Can you work these out from the model? Positions are in its coordinate system, mm. Face numbers are marked on the shaded views. A direction names the side the tool comes from. Give positions to 0.01 mm unless a question says otherwise; leave off trailing zeros. Order: outer loops, then holes, each group sorted by start corner. A loop starts at its lowest first (then second) coordinate and runs counter-clockwise, first axis right, second up.
Item 1: I'm going to push flat-ended pins straight in: pin 1 Ø6 at (x, y) = (63.5, 26.5) entering from -Z; pin 2 Ø10 at (x, y) = (108, 65) entering from +Z; pin 3 Ø10 at (x, y) = (104.5, 45.5) entering from -Z. Where does each tip first touch, or does it pass through?
Item 2: I want a section at C-C, the plane z = -7. Write out the boundary of the cut face in (x, y), then the cut area to 3 significant figures.
Item 3: Which directions (+Z, -Z, +X, -X, +Y, -Y) give clear straight access to the entire face, cutting with the end or side of a thin tool? Please do the marked faces 4, 5, 6, 7 and 8.
Item 4: I want a section at B-B, the plane y = 104.5. Write out the boundary of the cut face in (x, z), then the cut area to 3 significant figures.
Item 5: I want a section at A-A, the plane x = 110. Write out the boundary of the cut face in (y, z).
Item 6: If we mould it in two halves opening along Z, with no side actions, what happens to the marked faces 1, 2 and 3? For each: +Z half, -Z half, draft (parallel to the pull), parting line (faces both ways), or undercut.
Item 7: If I drill on line 1 along Z through (x, y) = (106.5, 78); line 2 along X through (y, z) = (33, -24.5); line 3 along X through (y, z) = (111.5, -23), over which ranges is the centre line in solid material (lowest first)?
```python
from build123d import *

# Parameters (mm, degrees)
BOSS_EXTRUDE1_DEPTH = 100
FILLET1_R           = 20
SKETCH5_W           = 40
SKETCH5_H           = 120
BOSS_EXTRUDE2_DEPTH = 20
SKETCH6_W           = 10
SKETCH6_H           = 30
CUT_EXTRUDE1_DEPTH  = 120
SKETCH7_W           = 100
SKETCH7_H           = 100
BOSS_EXTRUDE3_DEPTH = 2
BOSS_EXTRUDE4_DEPTH = 100
SKETCH11_W          = 0.49
SKETCH11_H          = 2
BOSS_EXTRUDE5_DEPTH = 100
SKETCH12_R          = 7.5
CUT_EXTRUDE2_DEPTH  = 40
SKETCH15_W          = 30
SKETCH15_H          = 50
BOSS_EXTRUDE6_DEPTH = 15
SKETCH16_W          = 15
SKETCH16_H          = 50
CUT_EXTRUDE3_DEPTH  = 10


with BuildPart() as part:
    # Sketch3 → Boss-Extrude1 (new body)
    with BuildSketch(Plane(origin=(0, 0, 0), x_dir=(1, 0, 0), z_dir=(0, 1, 0))):
        Polygon((0, 0), (100, 0), (100, 20), (70, 20), align=None)
    extrude(amount=BOSS_EXTRUDE1_DEPTH)

    # Fillet1
    fillet1_edges = [part.edges().sort_by_distance(p)[0] for p in [
        (70, 50, -20),
    ]]
    fillet(fillet1_edges, radius=FILLET1_R)

    # Sketch5 → Boss-Extrude2 (add)
    with BuildSketch(Plane(origin=(100, 0, 0), x_dir=(0, 0, -1), z_dir=(1, 0, 0))):
        with Locations((9.230478953, 50)):
            Rectangle(SKETCH5_W, SKETCH5_H)
    extrude(amount=BOSS_EXTRUDE2_DEPTH)

    # Sketch6 → Cut-Extrude1 (cut)
    with BuildSketch(Plane(origin=(0, 110, 0), x_dir=(1, 0, 0), z_dir=(0, 1, 0))):
        with Locations((110, 9.230478953)):
            Rectangle(SKETCH6_W, SKETCH6_H)
    extrude(amount=-CUT_EXTRUDE1_DEPTH, mode=Mode.SUBTRACT)

    # Sketch7 → Boss-Extrude3 (add)
    with BuildSketch(Plane.XY):
        with Locations((50, 50)):
            Rectangle(SKETCH7_W, SKETCH7_H)
    extrude(amount=BOSS_EXTRUDE3_DEPTH)

    # Sketch10 → Boss-Extrude4 (add)
    with BuildSketch(Plane(origin=(0, 100, 0), x_dir=(1, 0, 0), z_dir=(0, 1, 0))):
        Polygon((100, -2), (98, -2), (99, -3), align=None)
        Polygon((95.99, -2), (96.99, -3), (97.99, -2), align=None)
        Polygon((93.98, -2), (94.98, -3), (95.98, -2), align=None)
        Polygon((91.97, -2), (92.97, -3), (93.97, -2), align=None)
        Polygon((89.96, -2), (90.96, -3), (91.96, -2), align=None)
        Polygon((87.95, -2), (88.95, -3), (89.95, -2), align=None)
        Polygon((85.94, -2), (86.94, -3), (87.94, -2), align=None)
        Polygon((83.93, -2), (84.93, -3), (85.93, -2), align=None)
        Polygon((81.92, -2), (82.92, -3), (83.92, -2), align=None)
        Polygon((79.91, -2), (80.91, -3), (81.91, -2), align=None)
        Polygon((77.9, -2), (78.9, -3), (79.9, -2), align=None)
        Polygon((75.89, -2), (76.89, -3), (77.89, -2), align=None)
        Polygon((73.88, -2), (74.88, -3), (75.88, -2), align=None)
        Polygon((71.87, -2), (72.87, -3), (73.87, -2), align=None)
        Polygon((69.86, -2), (70.86, -3), (71.86, -2), align=None)
        Polygon((67.85, -2), (68.85, -3), (69.85, -2), align=None)
        Polygon((65.84, -2), (66.84, -3), (67.84, -2), align=None)
        Polygon((63.83, -2), (64.83, -3), (65.83, -2), align=None)
        Polygon((61.82, -2), (62.82, -3), (63.82, -2), align=None)
        Polygon((59.81, -2), (60.81, -3), (61.81, -2), align=None)
        Polygon((57.8, -2), (58.8, -3), (59.8, -2), align=None)
        Polygon((55.79, -2), (56.79, -3), (57.79, -2), align=None)
        Polygon((53.78, -2), (54.78, -3), (55.78, -2), align=None)
        Polygon((51.77, -2), (52.77, -3), (53.77, -2), align=None)
        Polygon((49.76, -2), (50.76, -3), (51.76, -2), align=None)
        Polygon((47.75, -2), (48.75, -3), (49.75, -2), align=None)
        Polygon((45.74, -2), (46.74, -3), (47.74, -2), align=None)
        Polygon((43.73, -2), (44.73, -3), (45.73, -2), align=None)
        Polygon((41.72, -2), (42.72, -3), (43.72, -2), align=None)
        Polygon((39.71, -2), (40.71, -3), (41.71, -2), align=None)
        Polygon((37.7, -2), (38.7, -3), (39.7, -2), align=None)
        Polygon((35.69, -2), (36.69, -3), (37.69, -2), align=None)
        Polygon((33.68, -2), (34.68, -3), (35.68, -2), align=None)
        Polygon((31.67, -2), (32.67, -3), (33.67, -2), align=None)
        Polygon((29.66, -2), (30.66, -3), (31.66, -2), align=None)
        Polygon((27.65, -2), (28.65, -3), (29.65, -2), align=None)
        Polygon((25.64, -2), (26.64, -3), (27.64, -2), align=None)
        Polygon((23.63, -2), (24.63, -3), (25.63, -2), align=None)
        Polygon((21.62, -2), (22.62, -3), (23.62, -2), align=None)
        Polygon((19.61, -2), (20.61, -3), (21.61, -2), align=None)
        Polygon((17.6, -2), (18.6, -3), (19.6, -2), align=None)
        Polygon((15.59, -2), (16.59, -3), (17.59, -2), align=None)
        Polygon((13.58, -2), (14.58, -3), (15.58, -2), align=None)
        Polygon((11.57, -2), (12.57, -3), (13.57, -2), align=None)
        Polygon((9.56, -2), (10.56, -3), (11.56, -2), align=None)
        Polygon((7.55, -2), (8.55, -3), (9.55, -2), align=None)
        Polygon((5.54, -2), (6.54, -3), (7.54, -2), align=None)
        Polygon((3.53, -2), (4.53, -3), (5.53, -2), align=None)
        Polygon((1.52, -2), (2.52, -3), (3.52, -2), align=None)
        Polygon((-0.49, -2), (0.51, -3), (1.51, -2), align=None)
    extrude(amount=-BOSS_EXTRUDE4_DEPTH)

    # Sketch11 → Boss-Extrude5 (add)
    with BuildSketch(Plane(origin=(0, 100, 0), x_dir=(1, 0, 0), z_dir=(0, 1, 0))):
        with Locations((-0.245, -1)):
            Rectangle(SKETCH11_W, SKETCH11_H)
    extrude(amount=-BOSS_EXTRUDE5_DEPTH)

    # Sketch12 → Cut-Extrude2 (cut)
    with BuildSketch(Plane.XY.offset(10.769521047)):
        with Locations((110, 10)):
            Circle(SKETCH12_R)
        with Locations((110, 90)):
            Circle(SKETCH12_R)
    extrude(amount=-CUT_EXTRUDE2_DEPTH, mode=Mode.SUBTRACT)

    # Sketch15 → Boss-Extrude6 (add)
    with BuildSketch(Plane(origin=(0, 110, 0), x_dir=(1, 0, 0), z_dir=(0, 1, 0))):
        with Locations((110, 9.230478953)):
            Rectangle(SKETCH15_W, SKETCH15_H)
    extrude(amount=BOSS_EXTRUDE6_DEPTH)

    # Sketch16 → Cut-Extrude3 (cut)
    with BuildSketch(Plane(origin=(0, 125, 0), x_dir=(1, 0, 0), z_dir=(0, 1, 0))):
        with Locations((110, 9.230478953)):
            Rectangle(SKETCH16_W, SKETCH16_H)
    extrude(amount=-CUT_EXTRUDE3_DEPTH, mode=Mode.SUBTRACT)


solid = part.part
```
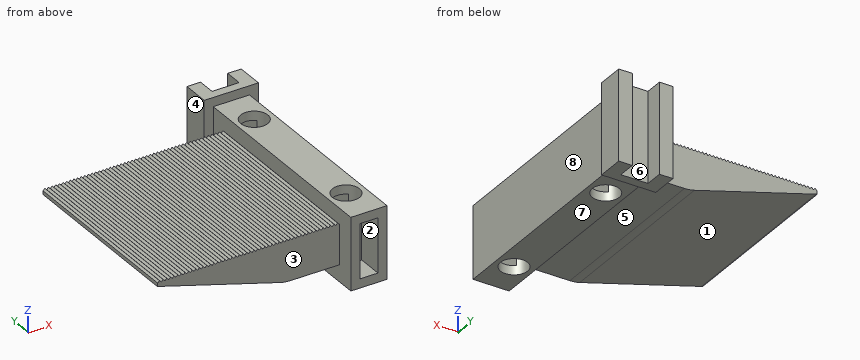
Results list:
1. pin 1: stops at z = -19
1. pin 2: stops at z = 10.77
1. pin 3: stops at z = -29.23
2. outline: (24.5, 0) - (100, 0) - (100, -10) - (105, -10) - (105, 4.41) arc R7.5 cw to (105, 15.59) - (105, 84.41) arc R7.5 cw to (105, 95.59) - (105, 110) - (115, 110) - (115, 95.59) arc R7.5 cw to (115, 84.41) - (115, 15.59) arc R7.5 cw to (115, 4.41) - (115, -10) - (120, -10) - (120, 110) - (125, 110) - (125, 125) - (117.5, 125) - (117.5, 115) - (102.5, 115) - (102.5, 125) - (95, 125) - (95, 110) - (100, 110) - (100, 100) - (24.5, 100) - close
2. area: 8,970 mm2
3. face 4: +Z, -Z, -X, +Y
3. face 5: -Z, -X, -Y
3. face 6: +Z, -Z, +Y
3. face 7: -Z, +X, -X, -Y
3. face 8: +Z, -Z, +X, -Y
4. outline: (100, -29.23) - (120, -29.23) - (120, 10.77) - (100, 10.77) - close; hole (105, -24.23) - (115, -24.23) - (115, 5.77) - (105, 5.77) - close
4. area: 500 mm2
5. outline: (-10, -29.23) - (2.5, -29.23) - (2.5, -24.23) - (-10, -24.23) - close; (-10, 5.77) - (2.5, 5.77) - (2.5, 10.77) - (-10, 10.77) - close; (17.5, -29.23) - (82.5, -29.23) - (82.5, -24.23) - (17.5, -24.23) - close; (17.5, 5.77) - (82.5, 5.77) - (82.5, 10.77) - (17.5, 10.77) - close; (97.5, -29.23) - (110, -29.23) - (110, -34.23) - (115, -34.23) - (115, 15.77) - (110, 15.77) - (110, 10.77) - (97.5, 10.77) - (97.5, 5.77) - (110, 5.77) - (110, -24.23) - (97.5, -24.23) - close
6. face 1: -Z half
6. face 2: undercut
6. face 3: draft
7. line 1: z = -29.23 to -24.23, 5.77 to 10.77
7. line 2: x = 100 to 120
7. line 3: x = 95 to 125
